Part model, mm, in its own coordinate system. A direction names the side the tool comes from. Give positions to 0.01 mm unless a question says otherwise; leave off trailing zeros. Loops run counter-clockwise (first coordinate to the right, second up) from the corner with the lowest first, then second, coordinate; pieces in that order, holes last. Notation, with made-up numbers: (44.5, 7) -> (48.5, 7) arc R15 ccw to (48.5, 18) -> close; hole circle Ø2 at (45.5, -27). An arc over 180 degrees is marked (long way). Write item = value, one per line.
from build123d import *

# Parameters (mm, degrees)
ESQUISSE1_R        = 2
BOSS_EXTRU_1_DEPTH = 4


with BuildPart() as part:
    # Esquisse1 → Boss.-Extru.1 (new body)
    with BuildSketch(Plane(origin=(0, 0, 0), x_dir=(1, 0, 0), z_dir=(0, 1, 0))):
        Polygon((0, 0), (28, 0), (0, -130), (28, -130), (28, -190), (172, -190), (172, -130), (200, -130), (172, 0), (200, 0), (200, 10), (0, 10), align=None)
        with Locations(Location((49.582205252, -147.769246608, 0), (0, 0, 270))):
            Circle(ESQUISSE1_R, mode=Mode.SUBTRACT)
        with Locations(Location((49.582205252, -171.460126827, 0), (0, 0, 270))):
            Circle(ESQUISSE1_R, mode=Mode.SUBTRACT)
        with Locations(Location((77.305575721, -18.22549733, 0), (0, 0, 270))):
            Circle(ESQUISSE1_R, mode=Mode.SUBTRACT)
        with Locations(Location((150.417794748, -171.460126827, 0), (0, 0, 90))):
            Circle(ESQUISSE1_R, mode=Mode.SUBTRACT)
        with Locations(Location((150.417794748, -147.769246608, 0), (0, 0, 90))):
            Circle(ESQUISSE1_R, mode=Mode.SUBTRACT)
        with Locations(Location((122.694424279, -18.22549733, 0), (0, 0, 90))):
            Circle(ESQUISSE1_R, mode=Mode.SUBTRACT)
        with BuildLine():
            Line((8.045765112, 6.656458485), (193.045765112, 6.656458485))
            ThreePointArc((193.045765112, 6.656458485), (194.702223597, 5), (193.045765112, 3.343541515))
            Line((193.045765112, 3.343541515), (8.045765112, 3.343541515))
            ThreePointArc((8.045765112, 3.343541515), (6.389306627, 5), (8.045765112, 6.656458485))
        make_face(mode=Mode.SUBTRACT)
    extrude(amount=BOSS_EXTRU_1_DEPTH)


solid = part.part
1) Slice it at C-C, the plane z = 165. List the corners of the cut face in (x, y).
Resolved:
outline = (28, 0) -> (172, 0) -> (172, 4) -> (28, 4) -> close
2) Slice it at A-A, the plane x = 142. List the corners of the cut face in (y, z).
Resolved:
outline = (0, -10) -> (4, -10) -> (4, -6.66) -> (0, -6.66) -> close; (0, -3.34) -> (4, -3.34) -> (4, 190) -> (0, 190) -> close
3) Drop flat-ended pins along their axis: P1, Ø3.5, axis at x = 49.58, z = 171.46, coming from the -Y side; P2, Ø2, axis at y = 3, z = 166.5, coming from the +X side; P3, Ø1.2, axis at x = 184, y = 3, coming from the +Z side; P4, Ø2, axis at y = 2, z = 147, coming from the -X side. Give the stop position or say it passes through.
Resolved:
P1 = through
P2 = 172
P3 = 130
P4 = 28
4) Drill centre lines: line 1 along Z through (x, y) = (49.5, 1.6); line 2 along X through (y, z) = (3.45, 148); line 3 along Z through (x, y) = (113, 1.2). Where is each one in solid material? Low to high. Write a range as [from, to].
Resolved:
line_1 = [-10, -6.66], [-3.34, 145.77], [149.77, 169.46], [173.46, 190]
line_2 = [28, 47.6], [51.57, 148.43], [152.4, 172]
line_3 = [-10, -6.66], [-3.34, 190]
5) Slice it at D-D, the plane z = 75.5. List the corners of the cut face in (x, y), and give its area (3 significant figures).
Resolved:
outline = (11.74, 0) -> (188.26, 0) -> (188.26, 4) -> (11.74, 4) -> close
area = 706 mm²
6) Slice it at B-B, the plane y = 2.75. List the corners of the cut face in (x, z), and give its area (3 significant figures).
Resolved:
outline = (0, -10) -> (200, -10) -> (200, 0) -> (172, 0) -> (200, 130) -> (172, 130) -> (172, 190) -> (28, 190) -> (28, 130) -> (0, 130) -> (28, 0) -> (0, 0) -> close; hole (8.05, -6.66) -> (193.05, -6.66) arc R1.66 ccw to (193.05, -3.34) -> (8.05, -3.34) arc R1.66 ccw to start; hole circle Ø4 at (49.58, 147.77); hole circle Ø4 at (49.58, 171.46); hole circle Ø4 at (77.31, 18.23); hole circle Ø4 at (122.69, 18.23); hole circle Ø4 at (150.42, 147.77); hole circle Ø4 at (150.42, 171.46)
area = 32,300 mm²
7) Which spindle directions (+Z, -Z, +X, -X, +Y, -Y) get a long thin tool onto all of the face, cutting with end or side? Do faces 1 (the face through (14.196, 1.972, 64.09)), 2 (the face through (186.196, 1.972, 65.91)), 3 (the face through (99, 0, 89)). Say none if no direction does.
Resolved:
face_1 = -X, +Y, -Y
face_2 = +X, +Y, -Y
face_3 = +Z, -Z, +X, -X, -Y
